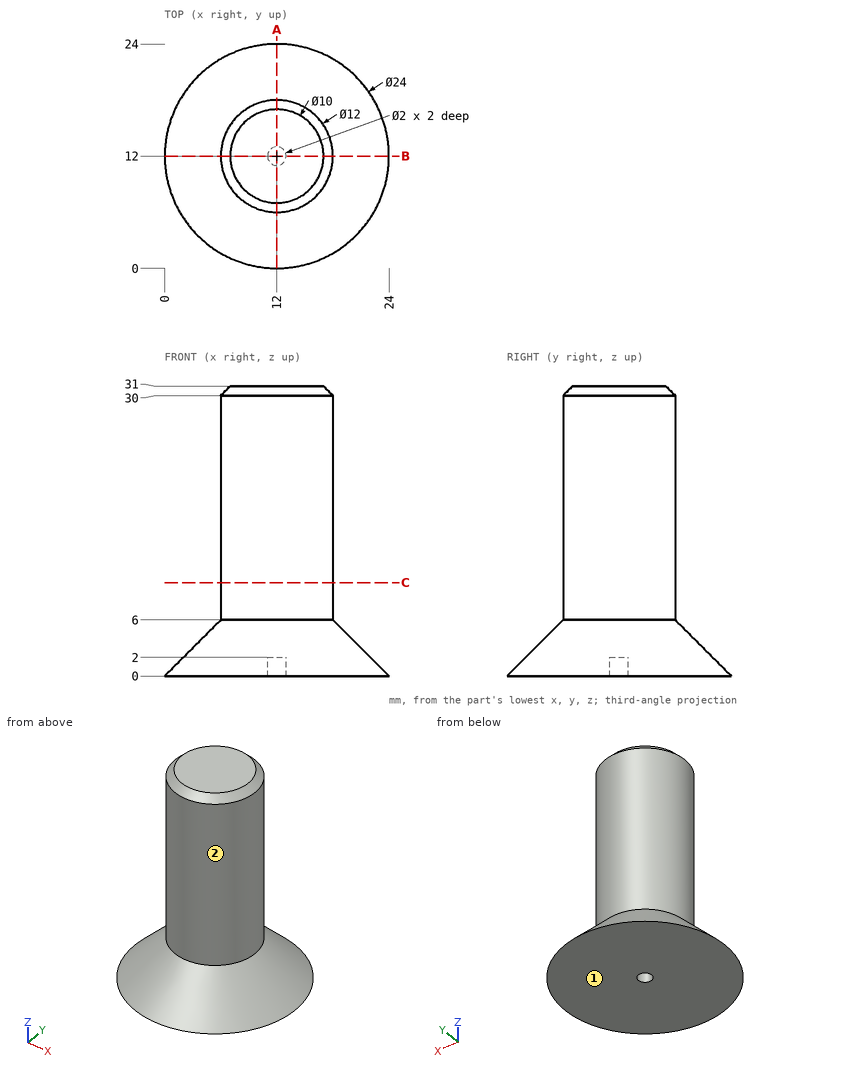
Study the drawing (mm; zero at the part's minimum x, y, z) and answer. A direction names the side the tool comes from. Coordinates: 2 decimals unless noted, no trailing zeros. Write each loop counter-clockwise with the first axis right and the second up, starting at its lowest first coordinate (ties: lowest second). Pieces come first, ordered by that corner, then holes. Notation, with made-up numbers: (66.5, 80) - (85.5, 80) arc R30 cw to (85.5, 106) - close; hole circle Ø4 at (87, 73.5). An arc over 180 degrees is marked (long way). Answer as a JSON object with one key per item and string values.
Q1. Which of the six approach directions +Z, -Z, +X, -X, +Y, -Y give full straight-line access (tool end or side, diameter ignored) to the marked faces 1 and 2?
Results list:
{"face 1": "-Z, +X, -X, +Y, -Y", "face 2": "+Z"}
Q2. Find section C-C (z = 10). Write down the section's boundary in (x, y), plus the area to 3 significant figures.
Results list:
{"outline": "circle Ø12 at (12, 12)", "area": "113 mm^2"}
Q3. Given pin 1 Ø1 at (x, y) = (12, 12) entering from -Z; pin 2 Ø1 at (x, z) = (15, 24) entering from -Y; pin 3 Ø12 at (x, z) = (7, 20) entering from -Y; pin 4 Ø3 at (x, y) = (11.5, 6) entering from +Z, each flat-ended and moving along its own axis, determine where each tip first touches the part or whether it passes through.
Results list:
{"pin 1": "stops at z = 2", "pin 2": "stops at y = 6.55", "pin 3": "stops at y = 6", "pin 4": "stops at z = 31"}
Q4. Consider L1, parallel to Y at x = 12, z = 1.35; L2, parallel to X at y = 12.25, z = 21; L3, parallel to X at y = 15.5, z = 3. Determine where each line is inside the solid, lowest interval first. Write a range as from..to.
Results list:
{"L1": "y = 1.35..11, 13..22.65", "L2": "x = 6.01..17.99", "L3": "x = 3.71..20.29"}
Q5. Find section A-A (x = 12). Write down the section's boundary in (y, z).
Results list:
{"outline": "(0, 0) - (11, 0) - (11, 2) - (13, 2) - (13, 0) - (24, 0) - (18, 6) - (18, 30) - (17, 31) - (7, 31) - (6, 30) - (6, 6) - close"}
